from build123d import *

# Parameters (mm, degrees)
SKETCH2_W           = 215.9
SKETCH2_H           = 114.3
SKETCH2_R           = 6.35
BOSS_EXTRUDE1_DEPTH = 19.05


with BuildPart() as part:
    # Sketch2 → Boss-Extrude1 (new body)
    with BuildSketch(Plane.XY):
        with Locations((359.786295427, 84.34467147)):
            Rectangle(SKETCH2_W, SKETCH2_H)
        with Locations(Location((277.236295427, 65.29467147, 0), (0, 0, 180))):
            Circle(SKETCH2_R, mode=Mode.SUBTRACT)
    extrude(amount=BOSS_EXTRUDE1_DEPTH)


solid = part.part
Source: CAD feature listing. Evaluate the final solid. Frame: model axes, mm. Give positions to 0.01 mm unless a question says otherwise; leave off trailing zeros. Write each loop counter-clockwise with the first axis right and the second up, starting at its lowest first coordinate (ties: lowest second). Pieces come first, ordered by that corner, then holes. Notation, with made-up numbers: (-9.5, 86) -> (-0.5, 86) arc R30 ccw to (-0.5, 119) -> close; hole circle Ø4 at (46, 39). An arc over 180 degrees is marked (long way). Return JSON: item names as keys, results as strings. Group by question number.
1. Section A-A, the plane y = 61.5. Output: boundary loops of the cut face in (x, z), then the cut area to 3 significant figures.
2. Section B-B, the plane x = 277.5. Output: boundary loops of the cut face in (y, z), then the cut area to 3 significant figures.
3. Mould query, pull axis X, two halves, no side actions, for faces 1 (the face through (251.836, 84, 9)), 2 (the face through (467.736, 84, 9)), 3 (the face through (274.31, 70.93, 9.39)), 4 (the face through (358, 85, 19.05)). Classes: +X half, -X half, draft (parallel to the pull), parting line (faces both ways), or undercut.
Determined:
{
 "1": {"outline": "(251.84, 0) -> (272.14, 0) -> (272.14, 19.05) -> (251.84, 19.05) -> close; (282.33, 0) -> (467.74, 0) -> (467.74, 19.05) -> (282.33, 19.05) -> close", "area": "3,920 mm2"},
 "2": {"outline": "(27.19, 0) -> (58.95, 0) -> (58.95, 19.05) -> (27.19, 19.05) -> close; (71.64, 0) -> (141.49, 0) -> (141.49, 19.05) -> (71.64, 19.05) -> close", "area": "1,940 mm2"},
 "3": {"face 1": "-X half", "face 2": "+X half", "face 3": "undercut", "face 4": "draft"}
}
